from build123d import *

# Parameters (mm, degrees)
SKETCH1_W         = 30
SKETCH1_H         = 159
CASE_2_DEPTH      = 97
CASE_SHELL_T      = 1
SKETCH2_R         = 2
PERFORATION_DEPTH = 1


with BuildPart() as part:
    # Sketch1 → Case 2 (new body)
    with BuildSketch(Plane.XY):
        with Locations((0, 79.5)):
            Rectangle(SKETCH1_W, SKETCH1_H)
    extrude(amount=CASE_2_DEPTH)

    # Case_shell (no face opened: a closed hollow body)
    add(offset(amount=-CASE_SHELL_T, mode=Mode.PRIVATE), mode=Mode.SUBTRACT)

    # Sketch2 → Perforation (cut)
    with BuildSketch(Plane.XY.offset(97)):
        with Locations((-9, 15)):
            Circle(SKETCH2_R)
        with Locations((-9, 21)):
            Circle(SKETCH2_R)
        with Locations((-9, 27)):
            Circle(SKETCH2_R)
        with Locations((-9, 33)):
            Circle(SKETCH2_R)
        with Locations((-9, 39)):
            Circle(SKETCH2_R)
        with Locations((-9, 45)):
            Circle(SKETCH2_R)
        with Locations((-9, 51)):
            Circle(SKETCH2_R)
        with Locations((-9, 57)):
            Circle(SKETCH2_R)
        with Locations((-9, 63)):
            Circle(SKETCH2_R)
        with Locations((-9, 69)):
            Circle(SKETCH2_R)
        with Locations((-9, 75)):
            Circle(SKETCH2_R)
        with Locations((-9, 81)):
            Circle(SKETCH2_R)
        with Locations((-9, 87)):
            Circle(SKETCH2_R)
        with Locations((-9, 93)):
            Circle(SKETCH2_R)
        with Locations((-9, 99)):
            Circle(SKETCH2_R)
        with Locations((-9, 105)):
            Circle(SKETCH2_R)
        with Locations((-9, 111)):
            Circle(SKETCH2_R)
        with Locations((-9, 117)):
            Circle(SKETCH2_R)
        with Locations((-9, 123)):
            Circle(SKETCH2_R)
        with Locations((-9, 129)):
            Circle(SKETCH2_R)
        with Locations((-9, 135)):
            Circle(SKETCH2_R)
        with Locations((-9, 141)):
            Circle(SKETCH2_R)
        with Locations((-3, 15)):
            Circle(SKETCH2_R)
        with Locations((-3, 21)):
            Circle(SKETCH2_R)
        with Locations((-3, 27)):
            Circle(SKETCH2_R)
        with Locations((-3, 33)):
            Circle(SKETCH2_R)
        with Locations((-3, 39)):
            Circle(SKETCH2_R)
        with Locations((-3, 45)):
            Circle(SKETCH2_R)
        with Locations((-3, 51)):
            Circle(SKETCH2_R)
        with Locations((-3, 57)):
            Circle(SKETCH2_R)
        with Locations((-3, 63)):
            Circle(SKETCH2_R)
        with Locations((-3, 69)):
            Circle(SKETCH2_R)
        with Locations((-3, 75)):
            Circle(SKETCH2_R)
        with Locations((-3, 81)):
            Circle(SKETCH2_R)
        with Locations((-3, 87)):
            Circle(SKETCH2_R)
        with Locations((-3, 93)):
            Circle(SKETCH2_R)
        with Locations((-3, 99)):
            Circle(SKETCH2_R)
        with Locations((-3, 105)):
            Circle(SKETCH2_R)
        with Locations((-3, 111)):
            Circle(SKETCH2_R)
        with Locations((-3, 117)):
            Circle(SKETCH2_R)
        with Locations((-3, 123)):
            Circle(SKETCH2_R)
        with Locations((-3, 129)):
            Circle(SKETCH2_R)
        with Locations((-3, 135)):
            Circle(SKETCH2_R)
        with Locations((-3, 141)):
            Circle(SKETCH2_R)
        with Locations((3, 15)):
            Circle(SKETCH2_R)
        with Locations((3, 21)):
            Circle(SKETCH2_R)
        with Locations((3, 27)):
            Circle(SKETCH2_R)
        with Locations((3, 33)):
            Circle(SKETCH2_R)
        with Locations((3, 39)):
            Circle(SKETCH2_R)
        with Locations((3, 45)):
            Circle(SKETCH2_R)
        with Locations((3, 51)):
            Circle(SKETCH2_R)
        with Locations((3, 57)):
            Circle(SKETCH2_R)
        with Locations((3, 63)):
            Circle(SKETCH2_R)
        with Locations((3, 69)):
            Circle(SKETCH2_R)
        with Locations((3, 75)):
            Circle(SKETCH2_R)
        with Locations((3, 81)):
            Circle(SKETCH2_R)
        with Locations((3, 87)):
            Circle(SKETCH2_R)
        with Locations((3, 93)):
            Circle(SKETCH2_R)
        with Locations((3, 99)):
            Circle(SKETCH2_R)
        with Locations((3, 105)):
            Circle(SKETCH2_R)
        with Locations((3, 111)):
            Circle(SKETCH2_R)
        with Locations((3, 117)):
            Circle(SKETCH2_R)
        with Locations((3, 123)):
            Circle(SKETCH2_R)
        with Locations((3, 129)):
            Circle(SKETCH2_R)
        with Locations((3, 135)):
            Circle(SKETCH2_R)
        with Locations((3, 141)):
            Circle(SKETCH2_R)
        with Locations((9, 15)):
            Circle(SKETCH2_R)
        with Locations((9, 21)):
            Circle(SKETCH2_R)
        with Locations((9, 27)):
            Circle(SKETCH2_R)
        with Locations((9, 33)):
            Circle(SKETCH2_R)
        with Locations((9, 39)):
            Circle(SKETCH2_R)
        with Locations((9, 45)):
            Circle(SKETCH2_R)
        with Locations((9, 51)):
            Circle(SKETCH2_R)
        with Locations((9, 57)):
            Circle(SKETCH2_R)
        with Locations((9, 63)):
            Circle(SKETCH2_R)
        with Locations((9, 69)):
            Circle(SKETCH2_R)
        with Locations((9, 75)):
            Circle(SKETCH2_R)
        with Locations((9, 81)):
            Circle(SKETCH2_R)
        with Locations((9, 87)):
            Circle(SKETCH2_R)
        with Locations((9, 93)):
            Circle(SKETCH2_R)
        with Locations((9, 99)):
            Circle(SKETCH2_R)
        with Locations((9, 105)):
            Circle(SKETCH2_R)
        with Locations((9, 111)):
            Circle(SKETCH2_R)
        with Locations((9, 117)):
            Circle(SKETCH2_R)
        with Locations((9, 123)):
            Circle(SKETCH2_R)
        with Locations((9, 129)):
            Circle(SKETCH2_R)
        with Locations((9, 135)):
            Circle(SKETCH2_R)
        with Locations((9, 141)):
            Circle(SKETCH2_R)
    extrude(amount=-PERFORATION_DEPTH, mode=Mode.SUBTRACT)


solid = part.part
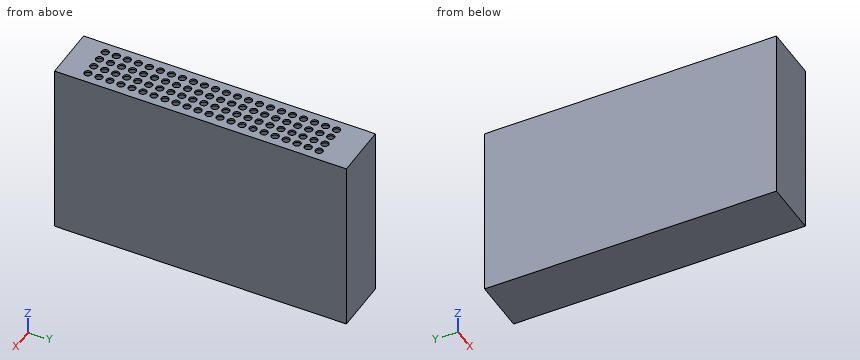
For this review, take the finished solid that the model builds, in its own axes (mm). Round coordinates to 2 decimals unless told otherwise and drop trailing zeros. Write each loop counter-clockwise with the first axis right and the second up, starting at its lowest first coordinate (ties: lowest second). Pieces come first, ordered by that corner, then holes. Notation, with made-up numbers: M 1,58 L 48,58 A29 ccw 48,81 Z; hole C 62,8 d7. An arc over 180 degrees is marked long. Write item = value, one per line. Start each with the question number.
(1) Clearance check with a flat-ended pin moving along its axis: pin 1 Ø2.5 at (x, y) = (9, 105) entering from +Z. State where the tip first meets the part, or that it passes through.
(2) We need section C-C (x = -3). Give the number of separate pieces and of enclosed holes in the cut face, then the cut area to 3 significant figures.
(3) We need section A-A (y = 135). Give the boundary of the cut face in (x, z), then the cut area to 3 significant figures.
(4) For line 1 along X through (y, z) = (26, 76); line 2 along Z through (x, y) = (6.75, 83.5); line 3 along X through (y, z) = (129, 96.7), list the stretches that pass through material, from the lowest coordinate up.
(5) We need section B-B (z = 59). Give the boundary of the cut face in (x, y).
Results found:
q1.pin_1 = 1
q2.separate_pieces = 22
q2.enclosed_holes = 0
q2.area = 420 mm²
q3.outline = M -15,0 L 15,0 L 15,97 L 11,97 L 11,96 L 14,96 L 14,1 L -14,1 L -14,96 L -11,96 L -11,97 L -15,97 Z; M -7,96 L -5,96 L -5,97 L -7,97 Z; M -1,96 L 1,96 L 1,97 L -1,97 Z; M 5,96 L 7,96 L 7,97 L 5,97 Z
q3.area = 234 mm²
q4.line_1 = -15 to -14, 14 to 15
q4.line_2 = 0 to 1, 96 to 97
q4.line_3 = -15 to -11, -7 to -5, -1 to 1, 5 to 7, 11 to 15
q5.outline = M -15,0 L 15,0 L 15,159 L -15,159 Z; hole M -14,1 L 14,1 L 14,158 L -14,158 Z
